```python
from build123d import *

# Parameters (mm, degrees)
BOX051_W                  = 0.9
BOX051_H                  = 8.1
BOX051_DEPTH              = 0.9
CHAMFER035_SIZE           = 0.89
BOX052_W                  = 0.9
BOX052_H                  = 8.1
BOX052_DEPTH              = 0.9
CHAMFER036_SIZE           = 0.89
BOX053_W                  = 0.8
BOX053_H                  = 2.2
BOX053_DEPTH              = 0.9
CHAMFER037_SIZE2          = 0.71
CHAMFER037_SIZE           = 0.89
BOX054_W                  = 0.8
BOX054_H                  = 2.2
BOX054_DEPTH              = 0.9
CHAMFER038_SIZE2          = 0.71
CHAMFER038_SIZE           = 0.89
BOX062_W                  = 0.9
BOX062_H                  = 6.4
BOX062_DEPTH              = 1.1
CHAMFER039_SIZE2          = 0.87
CHAMFER039_SIZE           = 1.09
BOX063_W                  = 0.9
BOX063_H                  = 6.4
BOX063_DEPTH              = 1.1
CHAMFER040_SIZE2          = 0.87
CHAMFER040_SIZE           = 1.09
CYLINDER017_R             = 0.4
CYLINDER017_DEPTH         = 0.8
CYLINDER018_R             = 0.4
CYLINDER018_DEPTH         = 0.8
CYLINDER019_R             = 0.4
CYLINDER019_DEPTH         = 0.7
CYLINDER020_R             = 0.4
CYLINDER020_DEPTH         = 0.7
BOX050_W                  = 10.2
BOX050_H                  = 3.8
BOX050_DEPTH              = 0.9
CHAMFER034_SIZE2          = 1.3
CHAMFER034_SIZE           = 0.4
FUSION015_PLACEMENT_ANGLE = 12


with BuildPart() as obj1:
    # Box051 → Box051 (new body)
    with BuildSketch(Plane(origin=(-6, -3.9, 1.6), x_dir=(1, 0, 0), z_dir=(0, 0, 1))):
        with Locations((0.45, 4.05)):
            Rectangle(BOX051_W, BOX051_H)
    extrude(amount=BOX051_DEPTH)

    # Chamfer035
    chamfer035_edges = [obj1.edges().sort_by_distance(p)[0] for p in [
        (-6, 4.2, 2.05),
    ]]
    chamfer(chamfer035_edges, length=CHAMFER035_SIZE)


with BuildPart() as obj2:
    # Box052 → Box052 (new body)
    with BuildSketch(Plane(origin=(5.1, -3.9, 1.6), x_dir=(1, 0, 0), z_dir=(0, 0, 1))):
        with Locations((0.45, 4.05)):
            Rectangle(BOX052_W, BOX052_H)
    extrude(amount=BOX052_DEPTH)

    # Chamfer036
    chamfer036_edges = [obj2.edges().sort_by_distance(p)[0] for p in [
        (6, 4.2, 2.05),
    ]]
    chamfer(chamfer036_edges, length=CHAMFER036_SIZE)


with BuildPart() as obj3:
    # Box053 → Box053 (new body)
    with BuildSketch(Plane(origin=(-5.1, 1, 1.6), x_dir=(1, 0, 0), z_dir=(0, 0, 1))):
        with Locations((0.4, 1.1)):
            Rectangle(BOX053_W, BOX053_H)
    extrude(amount=BOX053_DEPTH)

    # Chamfer037
    chamfer037_edges = [obj3.edges().sort_by_distance(p)[0] for p in [
        (-4.7, 1, 1.6),
    ]]
    chamfer037_side = obj3.faces().sort_by_distance((-4.7, 1, 2.05))[0]
    chamfer(chamfer037_edges, length=CHAMFER037_SIZE, length2=CHAMFER037_SIZE2, reference=chamfer037_side)


with BuildPart() as obj4:
    # Box054 → Box054 (new body)
    with BuildSketch(Plane(origin=(4.3, 1, 1.6), x_dir=(1, 0, 0), z_dir=(0, 0, 1))):
        with Locations((0.4, 1.1)):
            Rectangle(BOX054_W, BOX054_H)
    extrude(amount=BOX054_DEPTH)

    # Chamfer038
    chamfer038_edges = [obj4.edges().sort_by_distance(p)[0] for p in [
        (4.7, 1, 1.6),
    ]]
    chamfer038_side = obj4.faces().sort_by_distance((4.7, 1, 2.05))[0]
    chamfer(chamfer038_edges, length=CHAMFER038_SIZE, length2=CHAMFER038_SIZE2, reference=chamfer038_side)


with BuildPart() as obj5:
    # Box062 → Box062 (new body)
    with BuildSketch(Plane(origin=(-6, -3.9, 0.5), x_dir=(1, 0, 0), z_dir=(0, 0, 1))):
        with Locations((0.45, 3.2)):
            Rectangle(BOX062_W, BOX062_H)
    extrude(amount=BOX062_DEPTH)

    # Chamfer039
    chamfer039_edges = [obj5.edges().sort_by_distance(p)[0] for p in [
        (-5.55, 2.5, 0.5),
    ]]
    chamfer039_side = obj5.faces().sort_by_distance((-5.55, 2.5, 1.05))[0]
    chamfer(chamfer039_edges, length=CHAMFER039_SIZE, length2=CHAMFER039_SIZE2, reference=chamfer039_side)


with BuildPart() as obj6:
    # Box063 → Box063 (new body)
    with BuildSketch(Plane(origin=(5.1, -3.9, 0.5), x_dir=(1, 0, 0), z_dir=(0, 0, 1))):
        with Locations((0.45, 3.2)):
            Rectangle(BOX063_W, BOX063_H)
    extrude(amount=BOX063_DEPTH)

    # Chamfer040
    chamfer040_edges = [obj6.edges().sort_by_distance(p)[0] for p in [
        (5.55, 2.5, 0.5),
    ]]
    chamfer040_side = obj6.faces().sort_by_distance((5.55, 2.5, 1.05))[0]
    chamfer(chamfer040_edges, length=CHAMFER040_SIZE, length2=CHAMFER040_SIZE2, reference=chamfer040_side)


with BuildPart() as obj7:
    # Cylinder017 → Cylinder017 (new body)
    with BuildSketch(Plane(origin=(-6.8, -3.5, 0.9), x_dir=(0, 0, -1), z_dir=(1, 0, 0))):
        Circle(CYLINDER017_R)
    extrude(amount=CYLINDER017_DEPTH)


with BuildPart() as obj8:
    # Cylinder018 → Cylinder018 (new body)
    with BuildSketch(Plane(origin=(6, -3.5, 0.9), x_dir=(0, 0, -1), z_dir=(1, 0, 0))):
        Circle(CYLINDER018_R)
    extrude(amount=CYLINDER018_DEPTH)


with BuildPart() as obj9:
    # Cylinder019 → Cylinder019 (new body)
    with BuildSketch(Plane(origin=(-5.8, 5.6, 2.1), x_dir=(0, 0, -1), z_dir=(1, 0, 0))):
        Circle(CYLINDER019_R)
    extrude(amount=CYLINDER019_DEPTH)


with BuildPart() as obj10:
    # Cylinder020 → Cylinder020 (new body)
    with BuildSketch(Plane(origin=(5.1, 5.6, 2.1), x_dir=(0, 0, -1), z_dir=(1, 0, 0))):
        Circle(CYLINDER020_R)
    extrude(amount=CYLINDER020_DEPTH)


with BuildPart() as obj11:
    # Box050 → Box050 (new body)
    with BuildSketch(Plane(origin=(-5.1, 3.2, 1.6), x_dir=(1, 0, 0), z_dir=(0, 0, 1))):
        with Locations((5.1, 1.9)):
            Rectangle(BOX050_W, BOX050_H)
    extrude(amount=BOX050_DEPTH)

    # Chamfer034
    chamfer034_edges = [obj11.edges().sort_by_distance(p)[0] for p in [
        (0, 7, 2.5),
    ]]
    chamfer034_side = obj11.faces().sort_by_distance((0, 7, 2.05))[0]
    chamfer(chamfer034_edges, length=CHAMFER034_SIZE, length2=CHAMFER034_SIZE2, reference=chamfer034_side)

    # Fusion015: union obj1, obj2, obj3, obj4, obj5, obj6, obj7, obj8, obj9, obj10
    add(obj1.part)
    add(obj2.part)
    add(obj3.part)
    add(obj4.part)
    add(obj5.part)
    add(obj6.part)
    add(obj7.part)
    add(obj8.part)
    add(obj9.part)
    add(obj10.part)


with BuildPart() as obj11_1:
    # Fusion015 placement: moved
    add(obj11.part.moved(Location((0, 0, 0.769273))).rotate(Axis((0, 0, 0.769273), (1, 0, 0)), FUSION015_PLACEMENT_ANGLE))


solid = obj11_1.part
```
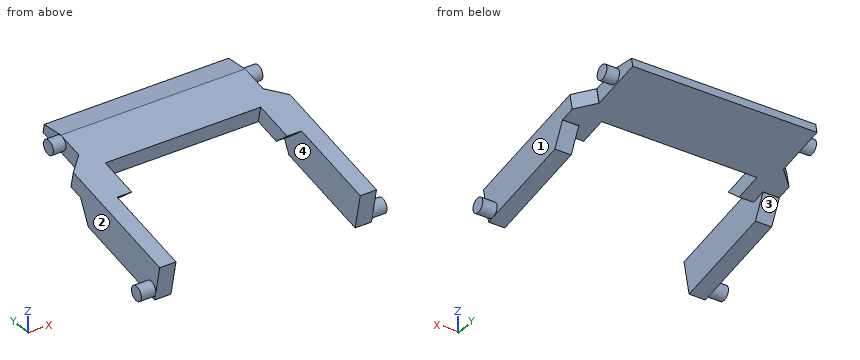
Part model, mm, in its own coordinate system. Face numbers are marked on the shaded views. Give positions to 0.01 mm unless a question says otherwise; leave off trailing zeros. Write each loop counter-clockwise with the first axis right and the second up, starting at its lowest first coordinate (ties: lowest second). Pieces come first, ordered by that corner, then holes. Notation, with made-up numbers: M 20.25,-13 L 43.25,-13 A20 cw 43.25,20 Z; hole C -9,88 d9. An arc over 180 degrees is marked long. Use CSV: the item, a comma, the result in double quotes.
Item 1: Slice it at C-C on x = -0.75. Write the cut outline in (y, z), plus the area to 3 significant figures.
Taken from the geometry:
outline,"M 2.61,3.88 L 2.8,3 L 6.51,3.79 L 6.41,4.28 L 5.06,4.4 Z"
area,"3.16 mm²"
Item 2: Slice it at B-B on z = 1.95. Write the cut outline in (x, y).
Taken from the geometry:
outline,"M -6,-4.24 L -5.1,-4.24 L -5.1,1.67 L -6,1.67 Z; M 5.1,-4.24 L 6,-4.24 L 6,1.67 L 5.1,1.67 Z"
Item 3: Pin check, flat tips, straight feed: P1, Ø1, axis at y = -1, z = 1.5, coming from the -X side; P2, Ø0.6, axis at y = 1.5, z = 3.5, coming from the +X side; P3, Ø0.9, axis at y = 5, z = 4, coming from the +X side. Stop position of each tip, or through.
Taken from the geometry:
P1,"stops at x = -6"
P2,"stops at x = 6"
P3,"stops at x = 5.8"
Item 4: Drill centre lines: probe 1 along X at (y, z) = (-2, 2.05); probe 2 along X at (y, z) = (3.75, 3.45); probe 3 along Z at (x, y) = (5.5, 1). Where is each one in solid material? Low to high.
Taken from the geometry:
probe 1,"x = -6 to -5.1, 5.1 to 6"
probe 2,"x = -5.1 to 5.1"
probe 3,"z = 1.49 to 3.54"
Item 5: Slice it at A-A on y = -0.25. Write the cut outline in (x, z).
Taken from the geometry:
outline,"M -6,1.23 L -5.1,1.23 L -5.1,3.27 L -6,3.27 Z; M 5.1,1.23 L 6,1.23 L 6,3.27 L 5.1,3.27 Z"
Item 6: Slice it at D-D on y = 1. Write the cut outline in (x, z).
Taken from the geometry:
outline,"M -6,1.49 L -5.1,1.49 L -5.1,2.97 L -4.3,2.97 L -4.3,3.54 L -6,3.54 Z; M 4.3,2.97 L 5.1,2.97 L 5.1,1.49 L 6,1.49 L 6,3.54 L 4.3,3.54 Z"
Item 7: Pull direction X, two halves, no side cores. Call the marked faces 1, 2, 3 and 4: +X half, -X half, draft (parallel to the pull), parting line (faces both ways), or undercut.
Taken from the geometry:
face 1,"+X half"
face 2,"-X half"
face 3,"draft"
face 4,"undercut"
